from build123d import *

# Parameters (mm, degrees)
BOSS_EXTRUDE1_DEPTH         = 4
BODY_MOVE_COPY2_ANGLE       = 180
SKETCH2_R                   = 9.5
BOSS_EXTRUDE2_DEPTH         = 153.4
BODY_MOVE_COPY3_START       = -613.6
BODY_MOVE_COPY3_OUTLINE_R   = 9.5
BODY_MOVE_COPY3_DEPTH       = 157.4
BODY_MOVE_COPY3_START_2     = -525.16
BODY_MOVE_COPY3_2_OUTLINE_R = 9.5
BODY_MOVE_COPY3_2_DEPTH     = 8
BODY_MOVE_COPY3_START_3     = -464.2
BODY_MOVE_COPY3_3_OUTLINE_R = 9.5
BODY_MOVE_COPY3_3_DEPTH     = 8
BODY_MOVE_COPY3_START_4     = -460.2
BODY_MOVE_COPY3_4_OUTLINE_R = 9.5
BODY_MOVE_COPY3_4_DEPTH     = 157.4
BODY_MOVE_COPY3_START_5     = -371.76
BODY_MOVE_COPY3_5_OUTLINE_R = 9.5
BODY_MOVE_COPY3_5_DEPTH     = 8
BODY_MOVE_COPY3_START_6     = -310.8
BODY_MOVE_COPY3_6_OUTLINE_R = 9.5
BODY_MOVE_COPY3_6_DEPTH     = 8
BODY_MOVE_COPY3_START_7     = -306.8
BODY_MOVE_COPY3_7_OUTLINE_R = 9.5
BODY_MOVE_COPY3_7_DEPTH     = 157.4
BODY_MOVE_COPY3_START_8     = -218.36
BODY_MOVE_COPY3_8_OUTLINE_R = 9.5
BODY_MOVE_COPY3_8_DEPTH     = 8
BODY_MOVE_COPY3_START_9     = -157.4
BODY_MOVE_COPY3_9_OUTLINE_R = 9.5
BODY_MOVE_COPY3_9_DEPTH     = 8
BODY_MOVE_COPY4_ANGLE       = 90
BODY_MOVE_COPY5_ANGLE       = 180
BODY_MOVE_COPY6_ANGLE       = 90
BOSS_EXTRUDE3_START         = 74.42
SKETCH2_2_R                 = 9.5
BOSS_EXTRUDE3_DEPTH         = 74.42
BOSS_EXTRUDE4_START         = -620.58
SKETCH2_3_R                 = 9.5
BOSS_EXTRUDE4_DEPTH         = 6.98


# Read off the part's stored shape, not the designer's step: Body-Move/Copy3
with BuildPart() as part:
    # Sketch1 → Boss-Extrude1 (new, symmetric)
    with BuildSketch(Plane(origin=(0, 0, 0), x_dir=(0, 0, -1), z_dir=(1, 0, 0))):
        with BuildLine():
            Line((5.499261314, 15.875), (10.998522628, 6.35))
            ThreePointArc((10.998522628, 6.35), (0, -12.7), (-10.998522628, 6.35))
            Line((-10.998522628, 6.35), (-5.499261314, 15.875))
            ThreePointArc((-5.499261314, 15.875), (0, 19.05), (5.499261314, 15.875))
        make_face()
    extrude(amount=BOSS_EXTRUDE1_DEPTH, both=True)


with BuildPart() as body_2:
    # Body-Move/Copy1: copy of part
    add(part.part.moved(Location((-60.96, 0, 0))))


with BuildPart() as body_2_1:
    # Body-Move/Copy2: moved
    add(body_2.part.rotate(Axis((0, 0, 0), (1, 0, 0)), BODY_MOVE_COPY2_ANGLE))


with BuildPart() as part_1:
    add(part.part)

    add(body_2_1.part)  # Boss-Extrude2 merges body 2
    # Sketch2 → Boss-Extrude2 (add)
    with BuildSketch(Plane(origin=(0, 0, 0), x_dir=(0, 0, -1), z_dir=(1, 0, 0))):
        Circle(SKETCH2_R)
    extrude(amount=-BOSS_EXTRUDE2_DEPTH)

    # Sketch2<2> → Boss-Extrude3 (add)
    with BuildSketch(Plane(origin=(0, 0, 0), x_dir=(0, 0, -1), z_dir=(1, 0, 0)).offset(BOSS_EXTRUDE3_START)):
        with Locations(Location((0, 0, 0), (0, 0, 180))):
            Circle(SKETCH2_2_R)
    extrude(amount=-BOSS_EXTRUDE3_DEPTH)


with BuildPart() as body_2_2:
    # Body-Move/Copy3 outline → Body-Move/Copy3 (new body)
    with BuildSketch(Plane.YZ.offset(BODY_MOVE_COPY3_START)):
        Circle(BODY_MOVE_COPY3_OUTLINE_R)
    extrude(amount=BODY_MOVE_COPY3_DEPTH)

    # Body-Move_Copy3 2 outline → Body-Move_Copy3 2 (add)
    with BuildSketch(Plane.YZ.offset(BODY_MOVE_COPY3_START_2)):
        with BuildLine():
            ThreePointArc((6.35, -10.998522628), (12.7, 0), (6.35, 10.998522628))
            ThreePointArc((6.35, 10.998522628), (0, 12.7), (-6.35, 10.998522628))
            Line((-6.35, 10.998522628), (-15.875, 5.499261314))
            ThreePointArc((-15.875, 5.499261314), (-19.05, 0), (-15.875, -5.499261314))
            Line((-15.875, -5.499261314), (-6.35, -10.998522628))
            ThreePointArc((-6.35, -10.998522628), (0, -12.7), (6.35, -10.998522628))
        make_face()
        Circle(BODY_MOVE_COPY3_2_OUTLINE_R, mode=Mode.SUBTRACT)
    extrude(amount=BODY_MOVE_COPY3_2_DEPTH)

    # Body-Move_Copy3 3 outline → Body-Move_Copy3 3 (add)
    with BuildSketch(Plane.YZ.offset(BODY_MOVE_COPY3_START_3)):
        with BuildLine():
            ThreePointArc((15.875, -5.499261314), (19.05, 0), (15.875, 5.499261314))
            Line((15.875, 5.499261314), (6.35, 10.998522628))
            ThreePointArc((6.35, 10.998522628), (-12.7, 0), (6.35, -10.998522628))
            Line((6.35, -10.998522628), (15.875, -5.499261314))
        make_face()
        Circle(BODY_MOVE_COPY3_3_OUTLINE_R, mode=Mode.SUBTRACT)
    extrude(amount=BODY_MOVE_COPY3_3_DEPTH)


with BuildPart() as body_3:
    # Body-Move_Copy3 4 outline → Body-Move_Copy3 4 (new body)
    with BuildSketch(Plane.YZ.offset(BODY_MOVE_COPY3_START_4)):
        Circle(BODY_MOVE_COPY3_4_OUTLINE_R)
    extrude(amount=BODY_MOVE_COPY3_4_DEPTH)

    # Body-Move_Copy3 5 outline → Body-Move_Copy3 5 (add)
    with BuildSketch(Plane.YZ.offset(BODY_MOVE_COPY3_START_5)):
        with BuildLine():
            ThreePointArc((6.35, -10.998522628), (12.7, 0), (6.35, 10.998522628))
            ThreePointArc((6.35, 10.998522628), (0, 12.7), (-6.35, 10.998522628))
            Line((-6.35, 10.998522628), (-15.875, 5.499261314))
            ThreePointArc((-15.875, 5.499261314), (-19.05, 0), (-15.875, -5.499261314))
            Line((-15.875, -5.499261314), (-6.35, -10.998522628))
            ThreePointArc((-6.35, -10.998522628), (0, -12.7), (6.35, -10.998522628))
        make_face()
        Circle(BODY_MOVE_COPY3_5_OUTLINE_R, mode=Mode.SUBTRACT)
    extrude(amount=BODY_MOVE_COPY3_5_DEPTH)

    # Body-Move_Copy3 6 outline → Body-Move_Copy3 6 (add)
    with BuildSketch(Plane.YZ.offset(BODY_MOVE_COPY3_START_6)):
        with BuildLine():
            ThreePointArc((15.875, -5.499261314), (19.05, 0), (15.875, 5.499261314))
            Line((15.875, 5.499261314), (6.35, 10.998522628))
            ThreePointArc((6.35, 10.998522628), (-12.7, 0), (6.35, -10.998522628))
            Line((6.35, -10.998522628), (15.875, -5.499261314))
        make_face()
        Circle(BODY_MOVE_COPY3_6_OUTLINE_R, mode=Mode.SUBTRACT)
    extrude(amount=BODY_MOVE_COPY3_6_DEPTH)


with BuildPart() as body_4:
    # Body-Move_Copy3 7 outline → Body-Move_Copy3 7 (new body)
    with BuildSketch(Plane.YZ.offset(BODY_MOVE_COPY3_START_7)):
        Circle(BODY_MOVE_COPY3_7_OUTLINE_R)
    extrude(amount=BODY_MOVE_COPY3_7_DEPTH)

    # Body-Move_Copy3 8 outline → Body-Move_Copy3 8 (add)
    with BuildSketch(Plane.YZ.offset(BODY_MOVE_COPY3_START_8)):
        with BuildLine():
            ThreePointArc((6.35, -10.998522628), (12.7, 0), (6.35, 10.998522628))
            ThreePointArc((6.35, 10.998522628), (0, 12.7), (-6.35, 10.998522628))
            Line((-6.35, 10.998522628), (-15.875, 5.499261314))
            ThreePointArc((-15.875, 5.499261314), (-19.05, 0), (-15.875, -5.499261314))
            Line((-15.875, -5.499261314), (-6.35, -10.998522628))
            ThreePointArc((-6.35, -10.998522628), (0, -12.7), (6.35, -10.998522628))
        make_face()
        Circle(BODY_MOVE_COPY3_8_OUTLINE_R, mode=Mode.SUBTRACT)
    extrude(amount=BODY_MOVE_COPY3_8_DEPTH)

    # Body-Move_Copy3 9 outline → Body-Move_Copy3 9 (add)
    with BuildSketch(Plane.YZ.offset(BODY_MOVE_COPY3_START_9)):
        with BuildLine():
            ThreePointArc((15.875, -5.499261314), (19.05, 0), (15.875, 5.499261314))
            Line((15.875, 5.499261314), (6.35, 10.998522628))
            ThreePointArc((6.35, 10.998522628), (-12.7, 0), (6.35, -10.998522628))
            Line((6.35, -10.998522628), (15.875, -5.499261314))
        make_face()
        Circle(BODY_MOVE_COPY3_9_OUTLINE_R, mode=Mode.SUBTRACT)
    extrude(amount=BODY_MOVE_COPY3_9_DEPTH)


with BuildPart() as body_4_1:
    # Body-Move/Copy4: moved
    add(body_4.part.rotate(Axis((0, 0, 0), (-1, 0, 0)), BODY_MOVE_COPY4_ANGLE))


with BuildPart() as body_3_1:
    # Body-Move/Copy5: moved
    add(body_3.part.rotate(Axis((0, 0, 0), (1, 0, 0)), BODY_MOVE_COPY5_ANGLE))


with BuildPart() as body_2_2_1:
    # Body-Move/Copy6: moved
    add(body_2_2.part.rotate(Axis((0, 0, 0), (1, 0, 0)), BODY_MOVE_COPY6_ANGLE))

    # Combine1: union part, body 4, body 3
    add(part_1.part)
    add(body_4_1.part)
    add(body_3_1.part)

    # Sketch2<3> → Boss-Extrude4 (add)
    with BuildSketch(Plane(origin=(0, 0, 0), x_dir=(0, 0, -1), z_dir=(1, 0, 0)).offset(BOSS_EXTRUDE4_START)):
        with Locations(Location((0, 0, 0), (0, 0, 90))):
            Circle(SKETCH2_3_R)
    extrude(amount=BOSS_EXTRUDE4_DEPTH)


solid = body_2_2_1.part
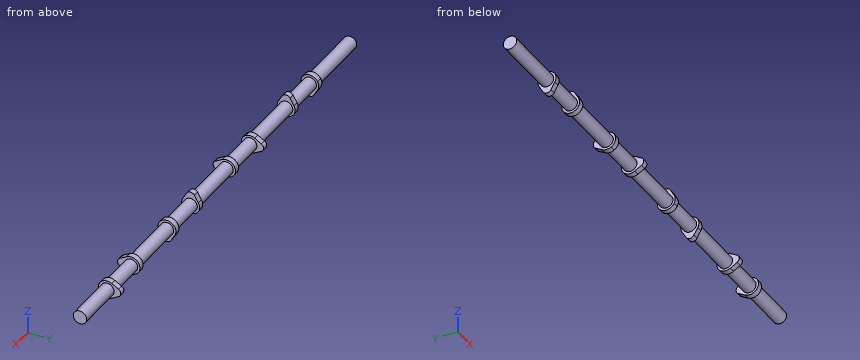
Build history of the part. All positions in model axes, mm. Round coordinates to 2 decimals unless told otherwise and drop trailing zeros. Write each loop counter-clockwise with the first axis right and the second up, starting at its lowest first coordinate (ties: lowest second). Pieces come first, ordered by that corner, then holes. Notation, with made-up numbers: (55.5, 70) - (72.5, 70) arc R14 cw to (72.5, 79) - close; hole circle Ø5 at (85, -30.5). An arc over 180 degrees is marked (long way). One line per question, with ' | ' between items.
1. Drop flat-ended pins along their axis: pin 1 Ø4 at (x, z) = (-305.5, -5.5) entering from -Y; pin 2 Ø6 at (y, z) = (-6, -11.5) entering from -X; pin 3 Ø5 at (x, y) = (-354, 12.5) entering from +Z; pin 4 Ø1 at (x, y) = (-500.5, -3.5) entering from -Z. Give the stop position or say it passes through.
Results are:
pin 1: y = -18 | pin 2: x = -525.16 | pin 3: through | pin 4: z = -9.01
2. Band-saw the part on A-A, the plane x = -337.5. Write the cut outline in (y, z), and give its area (3 significant figures).
Results are:
outline: circle Ø19 at (0, 0) | area: 284 mm^2
3. Drill centre lines: line 1 along X through (y, z) = (-8.5, 10); line 2 along Z through (x, y) = (-552, 7.5); line 3 along Y through (x, z) = (-153.5, -3). Where is each one in solid material? Low to high. Write a range as from..to.
Results are:
line 1: -464.2..-456.2, -218.36..-210.36 | line 2: -5.83..5.83 | line 3: -12.34..12.34
